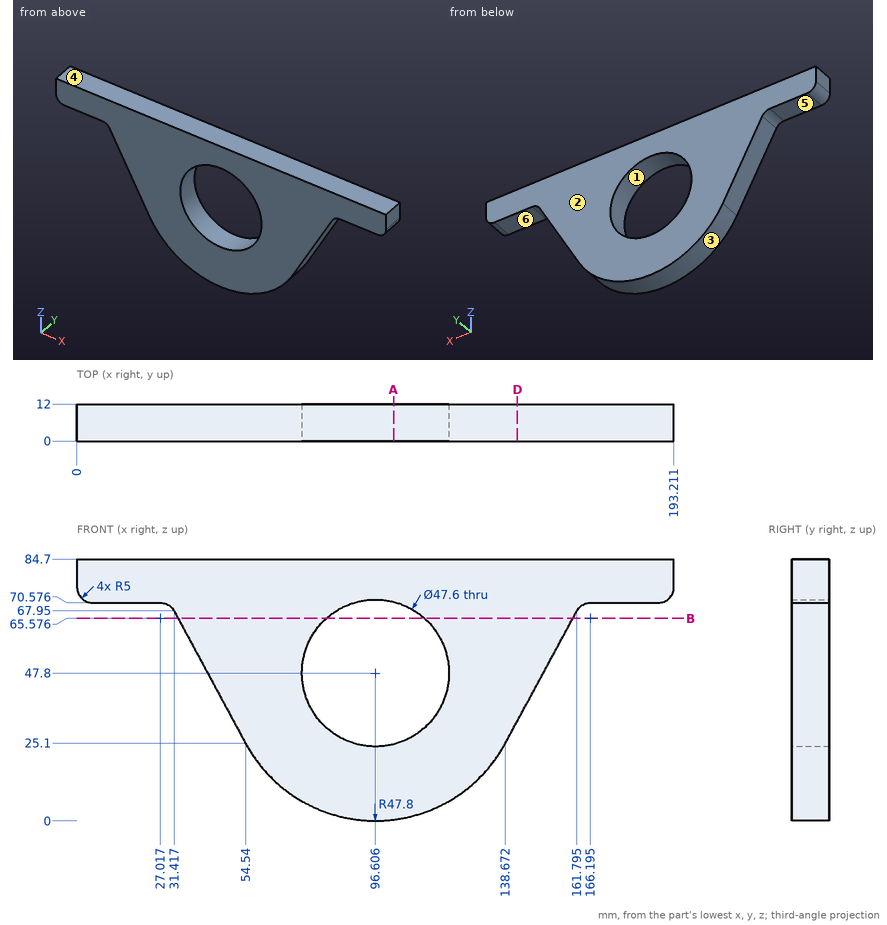
Design review of the part shown in the three views and the two pictorial views. Dimensions are in mm from the part's minimum x, y and z. A direction names the side the tool comes from. Round coordinates to 2 decimals unless told otherwise and drop trailing zeros. Order: outer loops, then holes, each group sorted by start corner. A loop starts at its lowest first (then second) coordinate and runs counter-clockwise, first axis right, second up.
Q1. Insertion check: P1, Ø6, axis at x = 182.5, y = 5, coming from the -Z side; P2, Ø4, axis at x = 118.5, y = 5.5, coming from the -Z side. Each pin has a flat end and moves straight along its axis. Give the tip position at first contact, or say it passes through.
Findings below:
P1: stops at z = 70.58
P2: stops at z = 4.34
Q2. Machinability: for the marked faces 4, 5 and 6, which of the approach directions +Z, -Z, +X, -X, +Y, -Y give a long, thin tool a straight path to every point of the face, cutting with its end or side? Answer none if there is none.
Findings below:
face 4: +Z, +X, -X, +Y, -Y
face 5: -Z, -X, +Y, -Y
face 6: -Z, +X, +Y, -Y
Q3. Wall thickness on line 1 (X direction, y = 10, z = 62) (1 decimal); line 2 (Z direction, x = 108.5, y = 9) (1 decimal); line 3 (X direction, y = 8.5, z = 27.5) (1 decimal): over which ranges is each line inside the solid? List them lowest first.
Findings below:
line 1: x = 34.6 to 77.5, 115.7 to 158.6
line 2: z = 1.5 to 27.2, 68.4 to 84.7
line 3: x = 53.2 to 84.2, 109 to 140
Q4. We need section D-D, the plane x = 142.5. Give the boundary of the cut face in (y, z) (1 decimal), plus the area to 3 significant figures.
Findings below:
outline: (0, 32.2) - (12, 32.2) - (12, 84.7) - (0, 84.7) - close
area: 630 mm2
Q5. We need section B-B, the plane z = 65.5. Give the boundary of the cut face in (x, y) (1 decimal), plus the area to 3 significant figures.
Findings below:
outline: (32.7, 0) - (80.7, 0) - (80.7, 12) - (32.7, 12) - close; (112.5, 0) - (160.5, 0) - (160.5, 12) - (112.5, 12) - close
area: 1,150 mm2
Q6. We need section A-A, the plane x = 102.5. Give the boundary of the cut face in (y, z) (1 decimal).
Findings below:
outline: (0, 0.4) - (12, 0.4) - (12, 24.7) - (0, 24.7) - close; (0, 70.9) - (12, 70.9) - (12, 84.7) - (0, 84.7) - close
Q7. Mouldability with a two-part tool opening along X and no side actions: class the marked faces 1, 2 and 3 as pulls with the +X half, pulls with the -X half, needs draft (parallel to the pull), parting line crosses it, or undercut.
Findings below:
face 1: undercut
face 2: needs draft
face 3: parting line crosses it
